Read the model definition and answer for the solid it produces. Units are mm, in the model's axes. Face numbers are marked on the shaded views. A direction names the side the tool comes from. Give positions to 0.01 mm unless a question says otherwise; leave off trailing zeros. Write each loop counter-clockwise with the first axis right and the second up, starting at its lowest first coordinate (ties: lowest second). Pieces come first, ordered by that corner, then holes. Notation, with made-up numbers: M 25,66.25 L 55,66.25 A15 cw 55,91.25 Z; hole C -20.5,9.5 d11. An arc over 180 degrees is marked long. Use a Markdown table: item, result. Add a question column.
Item 1: A cutting plane is placed at D-D on y = 48. Determine the outline of the cut face in (x, z), then the cut area to 3 significant figures.
Item 2: Consider probe 1 along Y at (x, z) = (-5, 8.5); probe 2 along Z at (x, y) = (-1.5, -27); probe 3 along Z at (x, y) = (-0.5, 21.5). Determine where each line is inside the solid, lowest interval first. Write a range as [from, to].
Item 3: For the marked faces 5, 6, 7, 8 and 9, determine the directions among +Z, -Z, +X, -X, +Y, -Y from which every point of the face is accessible in a straight line to the end or side of a thin tool.
Item 4: A cutting plane is placed at A-A on y = 10.5. Determine the outline of the cut face in (x, z).
Item 5: The mould has two halves that part along X. Classify the marked faces 1, 2, 3 and 4: pulls with the +X half, pulls with the -X half, needs draft (parallel to the pull), parting line crosses it, or undercut.
Item 6: A cutting plane is placed at B-B on x = 17. Determine the outline of the cut face in (y, z).
Item 7: A cutting plane is placed at C-C on z = 7.25. Count the separate pieces of the cut face and the enclosed holes in it, then the cut area to 3 significant figures.
Item 8: Given P1, Ø10, axis at x = 0.5, y = -18, coming from the -Z side; P2, Ø13, axis at x = 1.5, y = 40.5, coming from the +Z side; P3, Ø2, axis at x = 13.5, z = 14, coming from the -Y side; P4, Ø1, axis at y = 2.5, z = 12, coming from the -X side, each flat-ended and moving along its own axis, determine where each tip first touches the part or whether it passes through.
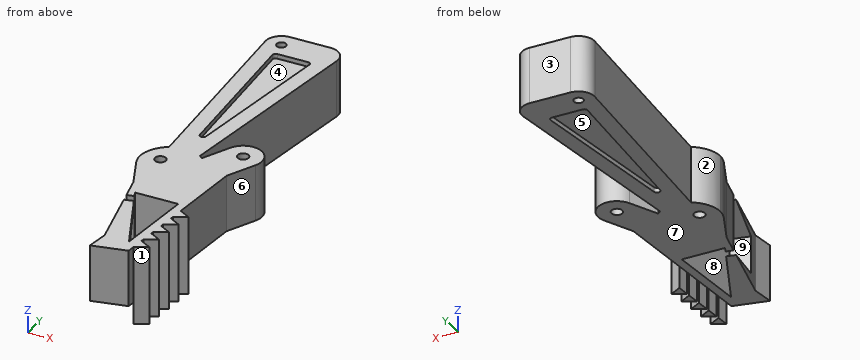
from build123d import *

# Parameters (mm, degrees)
BOSS_EXTRUDE1_DEPTH = 18
CUT_EXTRUDE1_DEPTH  = 25
BOSS_EXTRUDE2_DEPTH = 25
LPATTERN1_COUNT     = 5
LPATTERN1_PITCH     = 5
FILLET1_R           = 10
FILLET2_R           = 5
SKETCH6_R           = 1.5
CUT_EXTRUDE2_DEPTH  = 25
CUT_EXTRUDE3_DEPTH  = 8
SKETCH8_R           = 1.75
CUT_EXTRUDE4_DEPTH  = 61
SKETCH9_R           = 1.75
CUT_EXTRUDE5_DEPTH  = 25
CUT_EXTRUDE6_DEPTH  = 1.5


with BuildPart() as part:
    # Sketch1 → Boss-Extrude1 (new body)
    with BuildSketch(Plane.XY):
        with BuildLine():
            Line((2.499482963, -2.64043917), (12.810164454, 67.606908446))
            Line((12.810164454, 67.606908446), (-11.189835546, 67.606908446))
            Line((-11.189835546, 67.606908446), (-7.494565689, -2.295487655))
            Line((-7.494565689, -2.295487655), (-12.494565689, -2.295487655))
            Line((-12.494565689, -2.295487655), (-12.494565689, -12.295487655))
            Line((-12.494565689, -12.295487655), (-7.295314078, -24.210511057))
            Line((-7.295314078, -24.210511057), (-0.711849738, -54.210511057))
            Line((-0.711849738, -54.210511057), (-1.728395801, -61.136305893))
            Line((-1.728395801, -61.136305893), (9.271604199, -58.722368968))
            Line((9.271604199, -58.722368968), (14.26065829, -8.971898224))
            Line((14.26065829, -8.971898224), (18.725806397, -0.0241358))
            ThreePointArc((18.725806397, -0.0241358), (16.036237527, 8.023610308), (7.988491349, 5.334041648))
            Line((7.988491349, 5.334041648), (3.523343243, -3.613720776))
            Line((3.523343243, -3.613720776), (2.499482963, -2.64043917))
        make_face()
    extrude(amount=BOSS_EXTRUDE1_DEPTH)

    # Sketch4 → Cut-Extrude1 (cut)
    with BuildSketch(Plane(origin=(0, 0, 0), x_dir=(-1, 0, 0), z_dir=(0, 0, -1))):
        Polygon((-7.01051812, -54.210511057), (-9.517556755, -29.210511057), (4.20080561, -29.210511057), align=None)
    extrude(amount=-CUT_EXTRUDE1_DEPTH, mode=Mode.SUBTRACT)

    # Sketch5 → Boss-Extrude2 (add)
    with BuildSketch(Plane.XY.offset(18)):
        Polygon((9.523497192, -56.210511057), (9.924623374, -52.210511057), (13.440851715, -54.210511057), align=None)
    boss_extrude2 = extrude(amount=-BOSS_EXTRUDE2_DEPTH)

    # LPattern1: Boss-Extrude2 ×5
    with Locations(*[Vector(0.09978108182512832, 0.9950094148850086, 0) * (i * LPATTERN1_PITCH) for i in range(1, LPATTERN1_COUNT)]):
        add(boss_extrude2)

    # Fillet1
    # the kernel refuses this fillet: 10 mm, written as the material it takes off along each edge
    with BuildSketch(Plane(origin=(-12.494565689, -12.295487655, -5.216984474), x_dir=(0, 1, 0), z_dir=(0, 0, 1))) as fillet1_piece_1:
        with BuildLine():
            CenterArc((FILLET1_R * 0.208679378975, -FILLET1_R), FILLET1_R, 90, 23.574579649)
            Line((-FILLET1_R * 0.191263052627, -FILLET1_R * 0.0834597382526), (-FILLET1_R * 0.199261901259, -FILLET1_R * 0.0651289330176))
            Line((-FILLET1_R * 0.199261901259, -FILLET1_R * 0.0651289330176), (-FILLET1_R * 0.0041735875795, FILLET1_R * 0.02))
            Line((-FILLET1_R * 0.0041735875795, FILLET1_R * 0.02), (FILLET1_R * 0.208679378975, FILLET1_R * 0.02))
            Line((FILLET1_R * 0.208679378975, FILLET1_R * 0.02), (FILLET1_R * 0.208679378975, 0))
        make_face()
    extrude(amount=28.433968949, mode=Mode.SUBTRACT)
    with BuildSketch(Plane(origin=(-12.494565689, -2.295487655, -21.650635095), x_dir=(1, 0, 0), z_dir=(0, 0, 1))) as fillet1_piece_2:
        with BuildLine():
            CenterArc((10, -8.660254038), FILLET1_R, 120, 60)
            Line((0, -8.660254038), (-0.2, -8.660254038))
            Line((-0.2, -8.660254038), (-0.2, 0))
            Line((-0.2, 0), (0, 0.2))
            ThreePointArc((0, 0.2), (2.5, 0.2), (4.9, 0.173205081))
            Line((4.9, 0.173205081), (5, 0))
        make_face()
    extrude(amount=61.301270189, mode=Mode.SUBTRACT)

    # Fillet2
    fillet2_edges = [part.edges().sort_by_distance(p)[0] for p in [
        (-11.189835546, 67.606908446, 9),
        (12.810164454, 67.606908446, 9),
    ]]
    fillet(fillet2_edges, radius=FILLET2_R)

    # Sketch6 → Cut-Extrude2 (cut)
    with BuildSketch(Plane.XY.offset(18)):
        with Locations((-5.91853771, 62.606908446)):
            Circle(SKETCH6_R)
    extrude(amount=-CUT_EXTRUDE2_DEPTH, mode=Mode.SUBTRACT)

    # Sketch7 → Cut-Extrude3 (cut)
    with BuildSketch(Plane(origin=(-12.028992373, -2.639748078, 0), x_dir=(0, 0, 1), z_dir=(-0.9767573067708646, -0.21434822991974342, 0))):
        Polygon((-0.5, -29.584055917), (18.5, -29.584055917), (15, -48.14094063), (3, -48.14094063), align=None)
    extrude(amount=-CUT_EXTRUDE3_DEPTH, mode=Mode.SUBTRACT)

    # Sketch8 → Cut-Extrude4 (cut)
    with BuildSketch(Plane.XY.offset(18)):
        with Locations((13.357148803, 2.654952784)):
            Circle(SKETCH8_R)
    extrude(amount=-CUT_EXTRUDE4_DEPTH, mode=Mode.SUBTRACT)

    # Sketch9 → Cut-Extrude5 (cut)
    with BuildSketch(Plane(origin=(0, 0, 0), x_dir=(-1, 0, 0), z_dir=(0, 0, -1))):
        with Locations((6.452791989, -9.487217743)):
            Circle(SKETCH9_R)
    extrude(amount=-CUT_EXTRUDE5_DEPTH, mode=Mode.SUBTRACT)

    # Sketch10 → Cut-Extrude6 (cut)
    with BuildSketch(Plane(origin=(0, 0, 0), x_dir=(-1, 0, 0), z_dir=(0, 0, -1))):
        with BuildLine():
            Line((-5.131333655, 57.606908446), (4.599961749, 57.606908446))
            ThreePointArc((4.599961749, 57.606908446), (5.325492441, 57.295098257), (5.598567407, 56.554118877))
            Line((5.598567407, 56.554118877), (3.02178942, 7.809923601))
            ThreePointArc((3.02178942, 7.809923601), (2.069628089, 6.863792291), (1.033784499, 7.717492305))
            Line((1.033784499, 7.717492305), (-6.120732918, 56.46168758))
            ThreePointArc((-6.120732918, 56.46168758), (-5.888043926, 57.260658832), (-5.131333655, 57.606908446))
        make_face()
    cut_extrude6 = extrude(amount=-CUT_EXTRUDE6_DEPTH, mode=Mode.SUBTRACT)

    # Mirror1: Cut-Extrude6 across plane
    add(cut_extrude6.mirror(Plane(origin=(0, 0, 9), x_dir=(1, 0, 0), z_dir=(0, 0, -1))), mode=Mode.SUBTRACT)


solid = part.part
Filled in:
| question | item | result |
|---|---|---|
| 1 | outline | M -10.15,0 L -5.15,0 L -5.15,1.5 L 4.88,1.5 L 4.88,0 L 9.93,0 L 9.93,18 L 4.88,18 L 4.88,16.5 L -5.15,16.5 L -5.15,18 L -10.15,18 Z |
| 1 | area | 331 mm² |
| 2 | probe 1 | [-31.39, -10.46], [-8.51, 61.42], [63.79, 67.61] |
| 2 | probe 2 | [0, 18] |
| 2 | probe 3 | [1.5, 16.5] |
| 3 | face 5 | -Z |
| 3 | face 6 | +Z, -Z, +X |
| 3 | face 7 | -Z, -X, +Y |
| 3 | face 8 | +Z, -Z |
| 3 | face 9 | -X |
| 4 | outline | M -8.17,0 L -3.16,0 L -3.16,1.5 L -0.63,1.5 L -0.63,0 L 4.43,0 L 4.43,18 L -0.63,18 L -0.63,16.5 L -3.16,16.5 L -3.16,18 L -8.17,18 Z |
| 5 | face 1 | pulls with the +X half |
| 5 | face 2 | pulls with the -X half |
| 5 | face 3 | needs draft |
| 5 | face 4 | undercut |
| 6 | outline | M -3.48,0 L 7.42,0 L 7.42,18 L -3.48,18 Z |
| 7 | separate pieces | 1 |
| 7 | enclosed holes | 3 |
| 7 | area | 2,120 mm² |
| 8 | P1 | z = 0 |
| 8 | P2 | z = 18 |
| 8 | P3 | y = -54.69 |
| 8 | P4 | x = -7.77 |
